Model file for the job. Use its own axes, mm. Round coordinates to 2 decimals unless told otherwise and drop trailing zeros. Loops run counter-clockwise (first coordinate to the right, second up) from the corner with the lowest first, then second, coordinate; pieces in that order, holes last. Notation, with made-up numbers: M -27,-13.5 L 0,-13.5 A27 ccw 0,22.5 Z; hole C 37.25,-31 d4. An arc over 180 degrees is marked long. Use a Markdown table: item, result. Add a question column.
Item 1: Pin check, flat tips, straight feed: P1, Ø5, axis at y = 29, z = -5, coming from the -X side; P2, Ø5, axis at x = 10, y = 30, coming from the +Z side. Stop position of each tip, or through.
Item 2: Saw through at A-A on z = -20. Write the cut outline in (x, y).
Item 3: Saw through at D-D on y = 15. Write the cut outline in (x, z), then the cut area to 3 significant figures.
Item 4: Saw through at B-B on z = -3. Write the cut outline in (x, y).
Item 5: Two-plate mould, pull along X, no slides. Class faces 1 (the cylindrical face through (20, 10, -26)), 2 (the cylindrical face through (2.1, 17.7, -38.2)), 3 (the flat face through (0, 17, -20)): +X half, -X half, draft (parallel to the pull), parting line (faces both ways), or undercut.
Item 6: Wall check: L1, parallel to X at y = 12, z = -3; L2, parallel to Y at x = 31, z = -30; L3, parallel to X at y = 32, z = -38. Give the ranges that are in metal, low to high. Write a range as from..to.
Item 7: Saw through at C-C on y = 30. Write the cut outline in (x, z).
```python
from build123d import *

# Parameters (mm, degrees)
SKETCH1_W           = 40
SKETCH1_H           = 40
BOSS_EXTRUDE1_DEPTH = 45
SKETCH2_R           = 4
CUT_EXTRUDE1_DEPTH  = 45
SKETCH3_R           = 4
CUT_EXTRUDE2_DEPTH  = 45
SKETCH4_R           = 4
SKETCH4_R_2         = 1.5
CUT_EXTRUDE13_DEPTH = 45
SKETCH9_W           = 40
SKETCH9_H           = 10
CUT_EXTRUDE18_DEPTH = 45


with BuildPart() as part:
    # Sketch1 → Boss-Extrude1 (new body)
    with BuildSketch(Plane(origin=(0, 0, 0), x_dir=(1, 0, 0), z_dir=(0, 1, 0))):
        with Locations((20, 20)):
            Rectangle(SKETCH1_W, SKETCH1_H)
    extrude(amount=BOSS_EXTRUDE1_DEPTH)

    # Sketch2 → Cut-Extrude1 (cut)
    with BuildSketch(Plane.XY):
        with Locations((10, 30)):
            Circle(SKETCH2_R)
        with Locations((30, 30)):
            Circle(SKETCH2_R)
    extrude(amount=-CUT_EXTRUDE1_DEPTH, mode=Mode.SUBTRACT)

    # Sketch3 → Cut-Extrude2 (cut)
    with BuildSketch(Plane(origin=(40, 0, 0), x_dir=(0, 0, -1), z_dir=(1, 0, 0))):
        with Locations((10, 10)):
            Circle(SKETCH3_R)
        with Locations((30, 10)):
            Circle(SKETCH3_R)
    extrude(amount=-CUT_EXTRUDE2_DEPTH, mode=Mode.SUBTRACT)

    # Sketch4 → Cut-Extrude13 (cut)
    with BuildSketch(Plane(origin=(0, 45, 0), x_dir=(1, 0, 0), z_dir=(0, 1, 0))):
        with Locations(Location((20, 20, 0), (0, 0, 270))):
            Circle(SKETCH4_R)
        with Locations(Location((3, 3, 0), (0, 0, 270))):
            Circle(SKETCH4_R_2)
        with Locations(Location((3, 37, 0), (0, 0, 270))):
            Circle(SKETCH4_R_2)
        with Locations(Location((37, 37, 0), (0, 0, 270))):
            Circle(SKETCH4_R_2)
        with Locations(Location((37, 3, 0), (0, 0, 270))):
            Circle(SKETCH4_R_2)
    extrude(amount=-CUT_EXTRUDE13_DEPTH, mode=Mode.SUBTRACT)

    # Sketch9 → Cut-Extrude18 (cut)
    with BuildSketch(Plane.XY):
        with Locations((20, 40)):
            Rectangle(SKETCH9_W, SKETCH9_H)
    extrude(amount=-CUT_EXTRUDE18_DEPTH, mode=Mode.SUBTRACT)


solid = part.part
```
Entries:
| question | item | result |
|---|---|---|
| 1 | P1 | x = 0 |
| 1 | P2 | through |
| 2 | outline | M 0,0 L 16,0 L 16,35 L 0,35 Z; M 24,0 L 40,0 L 40,35 L 24,35 Z; hole C 10,30 d8; hole C 30,30 d8 |
| 3 | outline | M 0,-40 L 40,-40 L 40,0 L 0,0 Z; hole C 3,-37 d3; hole C 3,-3 d3; hole C 20,-20 d8; hole C 37,-37 d3; hole C 37,-3 d3 |
| 3 | area | 1,520 mm2 |
| 4 | outline | M 0,0 L 1.5,0 L 1.5,35 L 0,35 Z; M 4.5,0 L 35.5,0 L 35.5,35 L 4.5,35 Z; M 38.5,0 L 40,0 L 40,35 L 38.5,35 Z; hole C 10,30 d8; hole C 30,30 d8 |
| 5 | face 1 | draft |
| 5 | face 2 | undercut |
| 5 | face 3 | -X half |
| 6 | L1 | 0..1.5, 4.5..35.5, 38.5..40 |
| 6 | L2 | 0..6, 14..26.13, 33.87..35 |
| 6 | L3 | 0..1.88, 4.12..6.54, 13.46..26.54, 33.46..35.88, 38.12..40 |
| 7 | outline | M 0,-40 L 6,-40 L 6,0 L 0,0 Z; M 14,-40 L 26,-40 L 26,0 L 14,0 Z; M 34,-40 L 40,-40 L 40,0 L 34,0 Z; hole C 3,-37 d3; hole C 3,-3 d3; hole C 20,-20 d8; hole C 37,-37 d3; hole C 37,-3 d3 |
